Source: CAD feature listing. Evaluate the final solid. Frame: model axes, mm. A direction names the side the tool comes from. Round coordinates to 2 decimals unless told otherwise and drop trailing zeros. Order: outer loops, then holes, each group sorted by start corner. A loop starts at its lowest first (then second) coordinate and runs counter-clockwise, first axis right, second up. Notation, with made-up numbers: M 66.25,-14 L 116.25,-14 A16 cw 116.25,14 Z; hole C 53.25,79.5 d8. An arc over 180 degrees is marked long. Use one line per item in the form item = value. Start each with the question number.
Q1. Reachability of faces 1 (the flat face through (1, 42, -47)), 2 (the flat face through (43.5, 36, 1)), 3 (the cylindrical face through (24.75, 30.08, 48.52)) from +Z, -Z, +X, -X, +Y, -Y: full face, straight path, thin tool, end or side. Return the list, or none.
Q2. Contact query for flat-ended pins moving along their axis: pin 1 (2 mm diameter, centred on x = 26.5, y = 30, fed in from +Z); pin 2 (3.5 mm diameter, centred on x = 3, z = -49, fed in from +Y); pin 3 (3 mm diameter, centred on x = -13.5, y = 30, fed in from -Z); pin 4 (4 mm diameter, centred on x = 26.5, y = 68, fed in from +Z). Output: stop coordinate, or through.
Q3. Pull-direction query (X, two-part tool) for faces 4 (the flat face through (-46.5, 43, 1)), 5 (the flat face through (25, 85, 1)), 6 (the flat face through (-1, 42, 47)); classes: pulls with the +X half, pulls with the -X half, needs draft (parallel to the pull), parting line crosses it, or undercut.
Q4. Section A-A (x = -13.5). Return the cut outline in (y, z).
Q5. Section B-B (y = 30). Return the cut outline in (x, z), plus the area to 3 significant figures.
Q6. Section D-D (z = -31.5). Return the cut outline in (x, y).
Q7. Material intervals for probe 1 along Y at (x, z) = (26.5, 48.5); probe 2 along X at (y, z) = (68, 47.95); probe 3 along X at (y, z) = (10, -13.5), sorted ascending.
Q8. Section C-C (x = 12). Return the cut outline in (y, z).
Autodesk Inventor part; units mm, degrees
ref_plane "YZ Plane" through (0, 0, 0) normal (1, 0, 0) x (0, 1, 0)
ref_plane "XZ Plane" through (0, 0, 0) normal (0, 1, 0) x (-1, 0, 0)
ref_plane "XY Plane" through (0, 0, 0) normal (0, 0, 1) x (1, 0, 0)
sketch "Esquisse1" plane through (0, 0, 0) normal (0, 1, 0) x (-1, 0, 0)
  line L0 (-46.5, 50) -> (46.5, 50)
  line L1 (46.5, 50) -> (46.5, -50)
  line L2 (46.5, -50) -> (-46.5, -50)
  line L3 (-46.5, -50) -> (-46.5, 50)
  line L4 (-46.5, 50) -> (46.5, -50) construction
  line L5 (46.5, 50) -> (-46.5, -50) construction
  point P0 (0, 0)
  dimension "d0" = 100
  dimension "d1" = 93
extrude "Extrusion1" add sketch "Esquisse1" along normal blind 88
sketch "Esquisse2" plane through (0, 0, 0) normal (0, -1, 0) x (1, 0, 0)
  line L0 (-43.5, 47) -> (43.5, 47)
  line L1 (43.5, 47) -> (43.5, -47)
  line L2 (43.5, -47) -> (-43.5, -47)
  line L3 (-43.5, -47) -> (-43.5, 47)
  line L4 (-43.5, 47) -> (43.5, -47) construction
  line L5 (43.5, 47) -> (-43.5, -47) construction
  line L6 (46.5, 50) -> (46.5, -50)
  line L7 (-46.5, 50) -> (46.5, 50)
  point P0 (0, 0)
  dimension "d4" = 3
  dimension "d5" = 3
extrude "Extrusion2" cut sketch "Esquisse2" against normal blind 85
sketch "Esquisse3" plane through (-46.5, 0, 50) normal (0, 0, 1) x (1, 0, 0)
  line L0 (0, 88) -> (93, 88)
  line L1 (93, 88) -> (78, 88)
  line L2 (78, 88) -> (78, 73)
  line L3 (78, 73) -> (93, 73)
  line L4 (93, 73) -> (93, 88)
  point P0 (46.5, 0)
  dimension "d8" = 15
  dimension "d9" = 15
extrude "Extrusion3" cut sketch "Esquisse3" against normal up to surface (100 mm away)
sketch "Esquisse4" plane through (-46.5, 0, 50) normal (0, 0, 1) x (1, 0, 0)
  circle A0 centre (73, 68) radius 1.75
  circle A1 centre (33, 68) radius 1.75
  circle A2 centre (73, 30) radius 1.75
  circle A3 centre (33, 30) radius 1.75
  line L0 (93, 0) -> (93, 73)
  line L1 (0, 88) -> (78, 88)
  point P0 (46.5, 0)
  dimension "d12" = 40
  dimension "d13" = 3.5
  dimension "d14" = 3.5
  dimension "d15" = 3.5
  dimension "d16" = 3.5
  dimension "d17" = 40
  dimension "d18" = 0
  dimension "d19" = 0
  dimension "d20" = 38
  dimension "d21" = 20
  dimension "d22" = 20
  dimension "d23" = 0
extrude "Extrusion4" cut sketch "Esquisse4" against normal up to surface (3 mm away)
sketch "Esquisse5" plane through (46.5, 0, -50) normal (0, 0, -1) x (-1, 0, 0)
  circle A0 centre (66.8, 77) radius 2.1
  circle A1 centre (41.4, 77) radius 2.1
  circle A2 centre (11, 44.9) radius 2.1
  circle A3 centre (11, 7.4) radius 2.1
  line L0 (0, 0) -> (0, 73)
  line L1 (15, 88) -> (93, 88)
  line L2 (15, 88) -> (15, 73)
  line L3 (15, 73) -> (0, 73)
  circle A4 centre (83, 7.4) radius 2.1
  line L4 (93, 0) -> (93, 88)
  point P0 (46.5, 0)
  dimension "d26" = 4.2
  dimension "d27" = 4.2
  dimension "d28" = 4.2
  dimension "d29" = 4.2
  dimension "d30" = 11
  dimension "d31" = 0
  dimension "d32" = 11
  dimension "d33" = 0
  dimension "d34" = 37.5
  dimension "d35" = 25.4
  dimension "d36" = 26.4
  dimension "d37" = 28.1
  dimension "d38" = 4.2
  dimension "d39" = 0
  dimension "d40" = 10
extrude "Extrusion5" add sketch "Esquisse5" along normal blind 5.7
sketch "Esquisse6" plane through (-36.5, 7.4, -55.7) normal (0, 0, -1) x (-1, 0, 0)
  point P0 (-36.5, -7.4)
sketch "Esquisse7" plane through (-46.5, 0, 50) normal (0, 0, 1) x (1, 0, 0)
  line L0 (0, 88) -> (78, 88)
  line L1 (65, 88) -> (40, 88)
  line L2 (40, 88) -> (40, 79)
  line L3 (40, 79) -> (65, 79)
  line L4 (65, 79) -> (65, 88)
  line L5 (78, 73) -> (78, 88)
  point P0 (46.5, 0)
  point P1 (78, 80.5)
  point P2 (65, 83.5)
  dimension "d43" = 25
  dimension "d44" = 13
  dimension "d45" = 9
extrude "Extrusion6" cut sketch "Esquisse7" against normal up to surface (100 mm away)
properties part number "support_imu_Impression 3D"
Results list:
q1.face_1 = -Y
q1.face_2 = +Y, -Y
q1.face_3 = +Z
q2.pin_1 = -47
q2.pin_2 = 79
q2.pin_3 = -50
q2.pin_4 = 50
q3.face_4 = pulls with the -X half
q3.face_5 = needs draft
q3.face_6 = undercut
q4.outline = M 0,-50 L 88,-50 L 88,50 L 69.75,50 L 69.75,47 L 85,47 L 85,-47 L 0,-47 Z; M 0,47 L 28.25,47 L 28.25,50 L 0,50 Z; M 31.75,47 L 66.25,47 L 66.25,50 L 31.75,50 Z
q5.outline = M -46.5,-50 L 46.5,-50 L 46.5,50 L 28.25,50 L 28.25,47 L 43.5,47 L 43.5,-47 L -43.5,-47 L -43.5,47 L -15.25,47 L -15.25,50 L -46.5,50 Z; M -11.75,47 L 24.75,47 L 24.75,50 L -11.75,50 Z
q5.area = 1,100 mm2
q6.outline = M -46.5,0 L -43.5,0 L -43.5,85 L -6.5,85 L -6.5,88 L -46.5,88 Z; M 18.5,85 L 31.5,85 L 31.5,88 L 18.5,88 Z; M 43.5,0 L 46.5,0 L 46.5,73 L 43.5,73 Z
q7.probe_1 = 0 to 28.25, 31.75 to 66.25, 69.75 to 88
q7.probe_2 = -46.5 to -15.25, -11.75 to 24.75, 28.25 to 46.5
q7.probe_3 = -46.5 to -43.5, 43.5 to 46.5
q8.outline = M 0,-50 L 79,-50 L 79,-47 L 0,-47 Z; M 0,47 L 79,47 L 79,50 L 0,50 Z
